Verification items for the finished model (mm, model axes). A direction names the side the tool comes from. Round coordinates to 2 decimals unless told otherwise and drop trailing zeros. Order: outer loops, then holes, each group sorted by start corner. A loop starts at its lowest first (then second) coordinate and runs counter-clockwise, first axis right, second up. Notation, with made-up numbers: (-31, 71.25) -> (-17, 71.25) arc R23 cw to (-17, 83.25) -> close; hole circle Ø11 at (42.25, 34.5). An arc over 180 degrees is marked (long way). Return JSON: item names as keys, results as strings. Group by question number.
Item 1: Sectioned sample at D-D on x = 1. Give the number of separate pieces and of enclosed holes in the cut face, plus the area to 3 significant figures.
Item 2: Scan lines: probe 1 along Y at (x, z) = (0.15, -22.5); probe 2 along Z at (x, y) = (1, 54.5); probe 3 along Y at (x, z) = (0.55, 4.5). Record each from-to range of solid material in increasing order. Write a range as from..to.
Item 3: Access from +Z, -Z, +X, -X, +Y, -Y to the whole of each face (thin tool, end or side, straight path). Record for faces 4 (the flat face through (1, 18, -24.97)), 5 (the cylindrical face through (0.99, 32.35, 1.43)), 6 (the flat face through (0, 11, -12)), 7 (the flat face through (1, 58, -2)).
Item 4: Sectioned sample at C-C on y = -6. Record the cut outline in (x, z).
Item 5: Sectioned sample at A-A on z = 14. Record the cut outline in (x, y), plus the area to 3 significant figures.
Item 6: Sectioned sample at B-B on y = 20. Record the cut outline in (x, z), plus the area to 3 significant figures.
Item 7: Depth check by flat-ended pin: pin 1 Ø0.6 at (x, z) = (1, 25.5) entering from +Y. Enter the tip coordinate at first touch or a pass-through.
Item 8: Draft check along Y on faces 1 (the flat face through (1, 60.75, -18)), 2 (the flat face through (1, 16.75, 3)), 3 (the flat face through (1, -23.75, -1)). Enter one of: pulls with the +Y half, pulls with the -Y half, needs draft (parallel to the pull), parting line crosses it, or undercut.
```python
from build123d import *

# Parameters (mm, degrees)
F0_W     = 20
F0_H     = 2
F1_DEPTH = 2


with BuildPart() as f1:
    # F0 (on Right) → F1 (new body)
    with BuildSketch(Plane.YZ):
        with BuildLine():
            ThreePointArc((-23.75, -28), (-23.164214, -29.414214), (-21.75, -30))
            Line((-21.75, -30), (-18.5, -30))
            Line((-18.5, -30), (-18.5, -22))
            Line((-18.5, -22), (-16.5, -22))
            Line((-16.5, -22), (-16.5, -30))
            Line((-16.5, -30), (23.75, -30))
            Line((23.75, -30), (53.5, -30))
            Line((53.5, -30), (53.5, -22))
            Line((53.5, -22), (55.5, -22))
            Line((55.5, -22), (55.5, -30))
            Line((55.5, -30), (58.75, -30))
            ThreePointArc((58.75, -30), (60.164214, -29.414214), (60.75, -28))
            Line((60.75, -28), (60.75, -8))
            Line((60.75, -8), (64.188984, -8))
            ThreePointArc((64.188984, -8), (65.603197, -7.414214), (66.188984, -6))
            Line((66.188984, -6), (66.188984, -4))
            Line((66.188984, -4), (50.188984, -4))
            Line((50.188984, -4), (50.188984, -2))
            Line((50.188984, -2), (66.188984, -2))
            Line((66.188984, -2), (66.188984, 0))
            ThreePointArc((66.188984, 0), (65.603197, 1.414214), (64.188984, 2))
            Line((64.188984, 2), (33.75, 2))
            ThreePointArc((33.75, 2), (32.335786, 1.414214), (31.75, 0))
            Line((31.75, 0), (31.75, -14))
            ThreePointArc((31.75, -14), (30.285534, -17.535534), (26.75, -19))
            Line((26.75, -19), (21.75, -19))
            ThreePointArc((21.75, -19), (18.214466, -17.535534), (16.75, -14))
            Line((16.75, -14), (16.75, 20))
            Line((16.75, 20), (21.75, 20))
            ThreePointArc((21.75, 20), (23.164214, 20.585786), (23.75, 22))
            Line((23.75, 22), (23.75, 24))
            Line((23.75, 24), (4.75, 24))
            Line((4.75, 24), (4.75, 26))
            Line((4.75, 26), (23.75, 26))
            Line((23.75, 26), (23.75, 28.229252))
            ThreePointArc((23.75, 28.229252), (23.244291, 29.558573), (21.982906, 30.215645))
            ThreePointArc((21.982906, 30.215645), (1.369577, 31.495032), (-19.260146, 30.51488))
            ThreePointArc((-19.260146, 30.51488), (-22.461518, 28.891292), (-23.75, 25.540973))
            Line((-23.75, 25.540973), (-23.75, -28))
        make_face()
        with Locations((18.5, -25.970025)):
            Rectangle(F0_W, F0_H, mode=Mode.SUBTRACT)
        with BuildLine():
            ThreePointArc((-14.75, 15), (-13.285534, 18.535534), (-9.75, 20))
            Line((-9.75, 20), (6.75, 20))
            ThreePointArc((6.75, 20), (10.285534, 18.535534), (11.75, 15))
            Line((11.75, 15), (11.75, -10))
            Line((11.75, -10), (-4.75, -10))
            ThreePointArc((-4.75, -10), (-11.821068, -7.071068), (-14.75, 0))
            Line((-14.75, 0), (-14.75, 15))
        make_face(mode=Mode.SUBTRACT)
    extrude(amount=F1_DEPTH)


solid = f1.part
```
Recorded:
{
 "1": {"separate pieces": "1", "enclosed holes": "2", "area": "2,790 mm²"},
 "2": {"probe 1": "-23.75..-18.5, -16.5..53.5, 55.5..60.75", "probe 2": "-22..-4, -2..2", "probe 3": "-23.75..-14.75, 11.75..16.75"},
 "3": {"face 4": "+X, -X", "face 5": "+Z, +X, -X", "face 6": "+Z, -Z, -X, +Y, -Y", "face 7": "+X, -X, +Y"},
 "4": {"outline": "(0, -30) -> (2, -30) -> (2, -9.92) -> (0, -9.92) -> close; (0, 20) -> (2, 20) -> (2, 31.4) -> (0, 31.4) -> close"},
 "5": {"outline": "(0, -23.75) -> (2, -23.75) -> (2, -14.75) -> (0, -14.75) -> close; (0, 11.75) -> (2, 11.75) -> (2, 16.75) -> (0, 16.75) -> close", "area": "28.0 mm²"},
 "6": {"outline": "(0, -30) -> (2, -30) -> (2, -26.97) -> (0, -26.97) -> close; (0, -24.97) -> (2, -24.97) -> (2, -18.68) -> (0, -18.68) -> close; (0, 20) -> (2, 20) -> (2, 24) -> (0, 24) -> close; (0, 26) -> (2, 26) -> (2, 30.44) -> (0, 30.44) -> close", "area": "35.5 mm²"},
 "7": {"pin 1": "y = 4.75"},
 "8": {"face 1": "pulls with the +Y half", "face 2": "undercut", "face 3": "pulls with the -Y half"}
}
